Geometry check sheet. Reference: the model listing, model coordinates, mm. Face numbers are marked on the shaded views. A direction names the side the tool comes from. Give positions to 0.01 mm unless a question says otherwise; leave off trailing zeros. Order: outer loops, then holes, each group sorted by start corner. A loop starts at its lowest first (then second) coordinate and runs counter-clockwise, first axis right, second up.
```python
from build123d import *

# Parameters (mm, degrees)
SKETCH002_W     = 53.5
SKETCH002_H     = 30.5
SKETCH002_W_2   = 19.5
SKETCH002_H_2   = 18
SKETCH002_W_3   = 3
SKETCH002_H_3   = 3.6
PAD001_DEPTH    = 2
SKETCH003_W     = 2
SKETCH003_H     = 11.25
SKETCH003_H_2   = 18
PAD002_DEPTH    = 1.5
SKETCH004_W     = 5.75
SKETCH004_H     = 18
PAD003_DEPTH    = 2.75
SKETCH005_W     = 53.5
SKETCH005_H     = 30.5
SKETCH005_W_2   = 49.5
SKETCH005_H_2   = 26.5
PAD004_DEPTH    = 40
SKETCH006_W     = 10
SKETCH006_H     = 4
POCKET001_DEPTH = 2
SKETCH008_W     = 6.5
SKETCH008_H     = 2.5
POCKET002_DEPTH = 5
SKETCH010_W     = 5.75
SKETCH010_H     = 2.15
POCKET003_DEPTH = 5
POCKET005_DEPTH = 0.75
SKETCH014_W     = 10
SKETCH014_H     = 2
PAD009_DEPTH    = 1
PAD010_DEPTH    = 42
POCKET006_DEPTH = 40


with BuildPart() as part:
    # Sketch002 → Pad001 (new body)
    with BuildSketch(Plane(origin=(0, -7.25, 0), x_dir=(0, 0, -1), z_dir=(0, -1, 0))):
        Rectangle(SKETCH002_W, SKETCH002_H)
        with Locations((8.75, 0)):
            Rectangle(SKETCH002_W_2, SKETCH002_H_2, mode=Mode.SUBTRACT)
        with Locations((-21.25, 7.4)):
            Rectangle(SKETCH002_W_3, SKETCH002_H_3, mode=Mode.SUBTRACT)
        with Locations((-21.25, -7.4)):
            Rectangle(SKETCH002_W_3, SKETCH002_H_3, mode=Mode.SUBTRACT)
    extrude(amount=-PAD001_DEPTH)

    # Sketch003 (on Face18 of Pad001) → Pad002 (join)
    with BuildSketch(Plane(origin=(0, -5.25, 0), x_dir=(0, 0, -1), z_dir=(0, 1, 0))):
        with Locations((-13.15, 0)):
            Rectangle(SKETCH003_W, SKETCH003_H)
        with Locations((-8.9, 0)):
            Rectangle(SKETCH003_W, SKETCH003_H_2)
    extrude(amount=PAD002_DEPTH)

    # Sketch004 (on Face5 of Pad002) → Pad003 (join)
    with BuildSketch(Plane(origin=(0, -5.25, 0), x_dir=(0, 0, -1), z_dir=(0, 1, 0))):
        with Locations((21.375, 0)):
            Rectangle(SKETCH004_W, SKETCH004_H)
    extrude(amount=PAD003_DEPTH)

    # Sketch005 (on Face5 of Pad003) → Pad004 (join)
    with BuildSketch(Plane(origin=(0, -5.25, 0), x_dir=(0, 0, -1), z_dir=(0, 1, 0))):
        Rectangle(SKETCH005_W, SKETCH005_H)
        Rectangle(SKETCH005_W_2, SKETCH005_H_2, mode=Mode.SUBTRACT)
    extrude(amount=PAD004_DEPTH)

    # Sketch006 (on Face34 of Pad004) → Pocket001 (cut)
    with BuildSketch(Plane(origin=(0, -7.25, 26.75), x_dir=(-1, 0, 0), z_dir=(0, 0, 1))):
        with Locations((0, -4.5)):
            Rectangle(SKETCH006_W, SKETCH006_H)
    extrude(amount=-POCKET001_DEPTH, mode=Mode.SUBTRACT)

    # Sketch008 (on Face5 of Pocket001) → Pocket002 (cut)
    with BuildSketch(Plane(origin=(15.25, -7.25, 0), x_dir=(0, 0, 1), z_dir=(1, 0, 0))):
        with Locations((-15, -39)):
            Rectangle(SKETCH008_W, SKETCH008_H)
        with Locations((15, -39)):
            Rectangle(SKETCH008_W, SKETCH008_H)
    extrude(amount=-POCKET002_DEPTH, mode=Mode.SUBTRACT)

    # Sketch010 (on Face3 of Pocket002) → Pocket003 (cut)
    with BuildSketch(Plane(origin=(-15.25, -7.25, 0), x_dir=(0, 0, -1), z_dir=(-1, 0, 0))):
        with Locations((0, -40.925)):
            Rectangle(SKETCH010_W, SKETCH010_H)
    extrude(amount=-POCKET003_DEPTH, mode=Mode.SUBTRACT)

    # Sketch013 (on Face5 of Pocket003) → Pocket005 (cut)
    with BuildSketch(Plane(origin=(15.25, 9.75, -3), x_dir=(0, 0, -1), z_dir=(1, 0, 0))):
        with BuildLine():
            Line((-11.643274, 3.192533), (-11.643274, 15.192533))
            Line((-11.643274, 15.192533), (-2.143274, 15.192533))
            Line((-2.143274, 15.192533), (0.389061, 9.211163))
            Line((0.389061, 9.211163), (3.856726, 15.192533))
            Line((3.856726, 15.192533), (13.356726, 15.192533))
            Line((13.356726, 15.192533), (13.356726, -2.807467))
            Line((13.356726, -2.807467), (-11.643274, -2.807467))
            ThreePointArc((-19.356726, 0), (-15.747516, -2.083778), (-11.643274, -2.807467))
            Line((-19.356726, 0), (-15.5, 4.596267))
            ThreePointArc((-15.5, 4.596267), (-13.695395, 3.554378), (-11.643274, 3.192533))
        make_face()
        Polygon((-5.643274, 9.192533), (-5.643274, 3.192533), (-2.164809, 3.192533), align=None, mode=Mode.SUBTRACT)
        Polygon((7.313657, 9.192533), (7.313657, 3.192533), (3.835191, 3.192533), align=None, mode=Mode.SUBTRACT)
    extrude(amount=-POCKET005_DEPTH, mode=Mode.SUBTRACT)

    # Sketch014 (on Face51 of Pocket005) → Pad009 (join)
    with BuildSketch(Plane(origin=(0, -7.25, 24.75), x_dir=(1, 0, 0), z_dir=(0, 0, -1))):
        with Locations((0, -8)):
            Rectangle(SKETCH014_W, SKETCH014_H)
    extrude(amount=PAD009_DEPTH)

    # Sketch015 (on Face1 of Pad009) → Pad010 (join)
    with BuildSketch(Plane(origin=(0, -7.25, 0), x_dir=(0, 0, -1), z_dir=(0, -1, 0))):
        Polygon((26.75, -15.25), (3.25, -15.25), (7.75, -19.75), (26.75, -19.75), align=None)
    extrude(amount=-PAD010_DEPTH)

    # Sketch016 (on Face78 of Pad010) → Pocket006 (cut)
    with BuildSketch(Plane(origin=(0, 34.75, 0), x_dir=(0, 0, -1), z_dir=(0, 1, 0))):
        Polygon((26.75, 15.25), (26.75, 17.75), (8.578427, 17.75), (6.078427, 15.25), align=None)
    extrude(amount=-POCKET006_DEPTH, mode=Mode.SUBTRACT)


solid = part.part
```
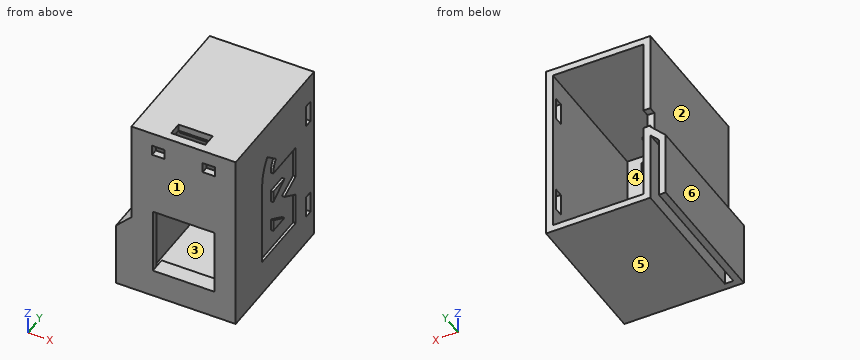
Q1. Thickness scan on L1, parallel to X at y = 23, z = -16; L2, parallel to X at y = 16, z = -20; L3, parallel to Z at x = -0.5, y = 21. Record the ranges inside material, lowest first.
Q2. Cross-section at C-C, the plane y = 29. Record the boundary of the cut face in (x, z), and give its area (3 significant figures).
Q3. Access from +Z, -Z, +X, -X, +Y, -Y to the whole of each face (thin tool, end or side, straight path). Record for the marked faces 1, 2 and 3.
Q4. Cross-section at D-D, the plane z = -23. Record the boundary of the cut face in (x, y).
Q5. Gauge pin test, flat ends, axial feed: P1, Ø8, axis at y = 1, z = 3.5, coming from the -X side; P2, Ø1.2, axis at x = 0.5, y = -4, coming from the +Z side; P3, Ø1.2, axis at x = -16.5, z = -12, coming from the +Y side. Record the tip position at first contact, or that the pin passes through.
Q6. Cross-section at B-B, the plane z = 17. Record the boundary of the cut face in (x, y).
Q7. Cross-section at A-A, the plane x = -7.5. Record the boundary of the cut face in (y, z).
Q8. Release check for a two-part mould opening along X. For the marked faces 4, 5 and 6 record: pulls with the +X half, pulls with the -X half, needs draft (parallel to the pull), parting line crosses it, or undercut.
Answers follow:
1. L1: x = -19.75 to -17.75, -15.25 to -13.25, 13.25 to 14.5
1. L2: x = -19.75 to -17.75, -15.25 to -13.25, 13.25 to 15.25
1. L3: z = -26.75 to -24.75, 24.75 to 26.75
2. outline: (-19.75, -26.75) - (-17.75, -26.75) - (-17.75, -8.58) - (-15.25, -6.08) - (-15.25, -26.75) - (15.25, -26.75) - (15.25, 26.75) - (-15.25, 26.75) - (-15.25, -3.25) - (-19.75, -7.75) - close; hole (-13.25, -24.75) - (13.25, -24.75) - (13.25, 24.75) - (-13.25, 24.75) - close
2. area: 367 mm2
3. face 1: +Z, -Z, +X, -X, -Y
3. face 2: +Z, -X, +Y, -Y
3. face 3: +Y
4. outline: (-19.75, -7.25) - (15.25, -7.25) - (15.25, 34.75) - (13.25, 34.75) - (13.25, -5.25) - (9, -5.25) - (9, -2.5) - (-9, -2.5) - (-9, -5.25) - (-13.25, -5.25) - (-13.25, 34.75) - (-15.25, 34.75) - (-15.25, -5.25) - (-17.75, -5.25) - (-17.75, 34.75) - (-19.75, 34.75) - close
5. P1: stops at x = -15.25
5. P2: stops at z = 14.15
5. P3: stops at y = -5.25
6. outline: (-15.25, -7.25) - (15.25, -7.25) - (15.25, 30.5) - (13.25, 30.5) - (13.25, -5.25) - (-13.25, -5.25) - (-13.25, 34.75) - (-15.25, 34.75) - close; (13.25, 33) - (15.25, 33) - (15.25, 34.75) - (13.25, 34.75) - close
7. outline: (-7.25, -26.75) - (34.75, -26.75) - (34.75, -24.75) - (-5.25, -24.75) - (-5.25, -24.25) - (-2.5, -24.25) - (-2.5, -18.5) - (-7.25, -18.5) - close; (-7.25, 1) - (-5.25, 1) - (-5.25, 7.9) - (-3.75, 7.9) - (-3.75, 9.9) - (-5.25, 9.9) - (-5.25, 19.75) - (-7.25, 19.75) - close; (-7.25, 22.75) - (-5.25, 22.75) - (-5.25, 24.75) - (34.75, 24.75) - (34.75, 26.75) - (-7.25, 26.75) - close
8. face 4: undercut
8. face 5: needs draft
8. face 6: pulls with the -X half
